The listing builds one solid part. Answer for the finished solid, in the listing's coordinates (mm). A direction names the side the tool comes from. Give positions to 0.01 mm unless a question says otherwise; leave off trailing zeros. Loops run counter-clockwise (first coordinate to the right, second up) from the corner with the lowest first, then second, coordinate; pieces in that order, holes last. Notation, with made-up numbers: M -1,21.25 L 32,21.25 A16 ccw 32,51.25 Z; hole C 21,86 d8. An arc over 180 degrees is marked long. One line per item, written item: value. Start each with the question number.
Q1. A cutting plane is placed at B-B, the plane y = 2.5. Determine the outline of the cut face in (x, z).
Q2. Consider L1, parallel to Z at x = 1, y = 2.75; L2, parallel to Y at x = 3.5, z = 40. Determine where each line is inside the solid, lowest interval first.
Q3. A cutting plane is placed at C-C, the plane z = 14. Determine the outline of the cut face in (x, y), and give its area (3 significant figures).
Q4. For faces 1 (the flat face through (0, 15, 22)), 2 (the flat face through (0, -2, 41)), determine the directions among +Z, -Z, +X, -X, +Y, -Y from which every point of the face is accessible in a straight line to the end or side of a thin tool.
Q5. Flat-ended cylindrical pins translate along their axes: pin 1 (3 mm diameter, centred on x = 15, z = 39, fed in from -Y); pin 2 (12 mm diameter, centred on x = 15, y = 3, fed in from -Z). Find the tip coordinate at first contact, or state that the pin passes through.
Q6. A cutting plane is placed at A-A, the plane x = -16. Determine the outline of the cut face in (y, z), and give its area (3 significant figures).
from build123d import *

# Parameters (mm, degrees)
SKETCH_1_W          = 40
SKETCH_1_H          = 30
EXTRUDE_1_DEPTH     = 45
SKETCH_6_W          = 41
SKETCH_6_H          = 26
CUT_EXTRUDE_1_DEPTH = 41
CHAMFER_1_SIZE      = 2


with BuildPart() as part:
    # 草图1 → 凸台-拉伸1 (new body)
    with BuildSketch(Plane.XY):
        Rectangle(SKETCH_1_W, SKETCH_1_H)
    extrude(amount=EXTRUDE_1_DEPTH)

    # 草图6 → 切除-拉伸1 (cut, through all)
    with BuildSketch(Plane.ZY.offset(20)):
        with Locations((20.5, -2)):
            Rectangle(SKETCH_6_W, SKETCH_6_H)
    extrude(amount=-CUT_EXTRUDE_1_DEPTH, mode=Mode.SUBTRACT)

    # 倒角1
    chamfer_1_edges = [part.edges().sort_by_distance(p)[0] for p in [
        (20, 13, 0),
        (-20, 13, 0),
        (20, -15, 43),
        (-20, -15, 43),
    ]]
    chamfer(chamfer_1_edges, length=CHAMFER_1_SIZE)


solid = part.part
Answer block:
1. outline: M -20,41 L 20,41 L 20,45 L -20,45 Z
2. L1: 41 to 45
2. L2: 11 to 15
3. outline: M -20,11 L 20,11 L 20,15 L -20,15 Z
3. area: 160 mm^2
4. face 1: +Z, -Z, +X, -X, +Y
4. face 2: -Z, +X, -X, -Y
5. pin 1: y = 11
5. pin 2: z = 41
6. outline: M -15,41 L 11,41 L 11,0 L 15,0 L 15,45 L -15,45 Z
6. area: 284 mm^2
